```python
from build123d import *

# Parameters (mm, degrees)
SKETCH_1_R                = 5
EXTRUDE_1_DEPTH           = 6
CUT_EXTRUDE_START         = -3
CUT_EXTRUDE_1_DEPTH       = 3
CUT_EXTRUDE_START_2       = -34
CUT_EXTRUDE_1_2_OUTLINE_R = 3
CUT_EXTRUDE_1_2_DEPTH     = 28


# Read off the part's stored shape, not the designer's step: ｶｯﾄ - 押し出し1
with BuildPart() as part:
    # ｽｹｯﾁ1 → ﾎﾞｽ - 押し出し1 (new body)
    with BuildSketch(Plane.XY):
        Circle(SKETCH_1_R)
    extrude(amount=EXTRUDE_1_DEPTH)

    # ｶｯﾄ - 押し出し1 outline → ｶｯﾄ - 押し出し1 (cut)
    with BuildSketch(Plane(origin=(0, 0, 0), x_dir=(-1, 0, 0), z_dir=(0, 0, -1)).offset(CUT_EXTRUDE_START)):
        Polygon((3.267510606, -0.936315364), (2.444628194, 2.36158951), (-0.822882412, 3.297904873), (-3.267510606, 0.936315364), (-2.444628194, -2.36158951), (0.822882412, -3.297904873), align=None)
    extrude(amount=CUT_EXTRUDE_1_DEPTH, mode=Mode.SUBTRACT)

    # Cut-Extrude 1 2 outline → Cut-Extrude 1 2 (add)
    with BuildSketch(Plane(origin=(0, 0, 0), x_dir=(-1, 0, 0), z_dir=(0, 0, -1)).offset(CUT_EXTRUDE_START_2)):
        Circle(CUT_EXTRUDE_1_2_OUTLINE_R)
    extrude(amount=CUT_EXTRUDE_1_2_DEPTH)


solid = part.part
```
CAD build for the part. Positions are in the model's coordinates, mm. A direction names the side the tool comes from. Round coordinates to 2 decimals unless told otherwise and drop trailing zeros. Order: outer loops, then holes, each group sorted by start corner. A loop starts at its lowest first (then second) coordinate and runs counter-clockwise, first axis right, second up. Notation, with made-up numbers: (57, 6.25) - (107, 6.25) arc R15 cw to (107, 31.25) - close; hole circle Ø8 at (-38.75, 48). An arc over 180 degrees is marked (long way). Answer as CSV lines item,"result". Start each with the question number.
1. Pin check, flat tips, straight feed: pin 1 (2 mm diameter, centred on x = 0, y = 0, fed in from -Z); pin 2 (4 mm diameter, centred on x = -0.5, y = 2.5, fed in from -Z); pin 3 (5 mm diameter, centred on y = -3, z = 6, fed in from -X); pin 4 (3 mm diameter, centred on x = -3, z = 6.5, fed in from -Y). Stop position of each tip, or through.
2. Saw through at D-D, the plane y = 3.75. Write the cut outline in (x, z), and give its area (3 significant figures).
3. Saw through at B-B, the plane z = 7. Write the cut outline in (x, y).
4. Pull direction Y, two halves, no side cores. Call faces 1 (the face through (0, 0, 34)), 2 (the face through (-1.08, -4.88, 2.96)), 3 (the face through (0, 0, 3)): +Y half, -Y half, draft (parallel to the pull), parting line (faces both ways), or undercut.
5. Drill centre lines: L1, parallel to X at y = 4, z = 3; L2, parallel to X at y = -1.75, z = 19; L3, parallel to Z at x = -2.5, y = -2.5. Where is each one in solid material? Low to high. Write a range as [from, to].
6. Saw through at C-C, the plane x = 0.5. Write the cut outline in (y, z).
7. Saw through at A-A, the plane y = 1.25. Write the cut outline in (x, z).
8. Tool access for faces 4 (the face through (2.86, -0.69, 1.52)), 5 (the face through (-0.1, -3.3, 6)), 6 (the face through (-0.1, -3.3, 0)): list every direction of +Z, -Z, +X, -X, +Y, -Y with a clear straight run to the whole face (end or side of a thin tool).
Model answer:
1,pin 1,"stops at z = 3"
1,pin 2,"stops at z = 0"
1,pin 3,"stops at x = -4.97"
1,pin 4,"stops at y = -4.74"
2,outline,"(-3.31, 0) - (3.31, 0) - (3.31, 6) - (-3.31, 6) - close"
2,area,"39.7 mm²"
3,outline,"circle Ø6 at (0, 0)"
4,face 1,"draft"
4,face 2,"parting line"
4,face 3,"undercut"
5,L1,"x = [-3, 3]"
5,L2,"x = [-2.44, 2.44]"
5,L3,"z = [0, 6]"
6,outline,"(-4.97, 0) - (-2.92, 0) - (-2.92, 3) - (3.21, 3) - (3.21, 0) - (4.97, 0) - (4.97, 6) - (2.96, 6) - (2.96, 34) - (-2.96, 34) - (-2.96, 6) - (-4.97, 6) - close"
7,outline,"(-4.84, 0) - (-2.72, 0) - (-2.72, 3) - (2.94, 3) - (2.94, 0) - (4.84, 0) - (4.84, 6) - (2.73, 6) - (2.73, 34) - (-2.73, 34) - (-2.73, 6) - (-4.84, 6) - close"
8,face 4,"-Z"
8,face 5,"+Z"
8,face 6,"-Z, +X, -X, +Y, -Y"
